from build123d import *

# Parameters (mm, degrees)
SKETCH1_W           = 8.482282434
SKETCH1_H           = 31.931379298
SKETCH1_R           = 3
SKETCH1_W_2         = 15
SKETCH1_H_2         = 6.200324761
SKETCH1_R_2         = 1.425
BOSS_EXTRUDE1_DEPTH = 4
FILLET3_R           = 25
FILLET4_R           = 5


with BuildPart() as part:
    # Sketch1 → Boss-Extrude1 (new body)
    with BuildSketch(Plane.XY):
        with BuildLine():
            ThreePointArc((4.241141217, 39.891935908), (0, 41.554196678), (-4.241141217, 39.891935908))
            Line((-4.241141217, 39.891935908), (-10, 28.882352941))
            Line((-10, 28.882352941), (-10, 0))
            Line((-10, 0), (-25.107692308, 0))
            Line((-25.107692308, 0), (-34, -17))
            Line((-34, -17), (34, -17))
            Line((34, -17), (25.107692308, 0))
            Line((25.107692308, 0), (10, 0))
            Line((10, 0), (10, 28.882352941))
            Line((10, 28.882352941), (4.241141217, 39.891935908))
        make_face()
        with Locations((0, 11.439217567)):
            Rectangle(SKETCH1_W, SKETCH1_H, mode=Mode.SUBTRACT)
        with Locations((0, 33)):
            Circle(SKETCH1_R, mode=Mode.SUBTRACT)
        with Locations((16.5, -5.259184167)):
            Rectangle(SKETCH1_W_2, SKETCH1_H_2, mode=Mode.SUBTRACT)
        with Locations((24, -12)):
            Circle(SKETCH1_R_2, mode=Mode.SUBTRACT)
        with Locations((-24, -12)):
            Circle(SKETCH1_R_2, mode=Mode.SUBTRACT)
        with Locations((-16.5, -5.259184167)):
            Rectangle(SKETCH1_W_2, SKETCH1_H_2, mode=Mode.SUBTRACT)
        with Locations((0, -12)):
            Circle(SKETCH1_R_2, mode=Mode.SUBTRACT)
    extrude(amount=BOSS_EXTRUDE1_DEPTH)

    # Fillet3
    # the kernel refuses this fillet: 25 mm, written as the material it adds along each edge
    with BuildSketch(Plane(origin=(10, 0, 0), x_dir=(1, 0, 0), z_dir=(0, 0, 1))) as fillet3_piece_1:
        with BuildLine():
            CenterArc((25, 22.959578579), FILLET3_R, 180, 66.690841486)
            Line((0, 22.959578579), (-0.5, 22.959578579))
            Line((-0.5, 22.959578579), (-0.5, 0))
            Line((-0.5, 0), (0, -0.5))
            ThreePointArc((0, -0.5), (7.553846154, -0.5), (14.909846154, -0.459191572))
            Line((14.909846154, -0.459191572), (15.107692308, 0))
        make_face()
    extrude(amount=4)
    with BuildSketch(Plane(origin=(-10, 0, 0), x_dir=(0, 1, 0), z_dir=(0, 0, 1))) as fillet3_piece_2:
        with BuildLine():
            CenterArc((22.959578579, 25), FILLET3_R, 203.309158514, 66.690841486)
            Line((0, 15.107692308), (-0.459191572, 14.909846154))
            ThreePointArc((-0.459191572, 14.909846154), (-0.5, 7.553846154), (-0.5, 0))
            Line((-0.5, 0), (0, -0.5))
            Line((0, -0.5), (22.959578579, -0.5))
            Line((22.959578579, -0.5), (22.959578579, 0))
        make_face()
    extrude(amount=4)

    # Fillet4
    # the kernel refuses this fillet: 5 mm, written as the material it adds along each edge
    with BuildSketch(Plane(origin=(4.241141217, -4.526472082, 0), x_dir=(0, 1, 0), z_dir=(0, 0, 1)), Plane(origin=(4.241141217, 27.404907216, 0), x_dir=(-1, 0, 0), z_dir=(0, 0, 1)), Plane(origin=(-24, -2.159021786, 0), x_dir=(0, -1, 0), z_dir=(0, 0, 1)), Plane(origin=(-9, -2.159021786, 0), x_dir=(-1, 0, 0), z_dir=(0, 0, 1)), Plane(origin=(9, -8.359346547, 0), x_dir=(1, 0, 0), z_dir=(0, 0, 1)), Plane(origin=(9, -2.159021786, 0), x_dir=(0, -1, 0), z_dir=(0, 0, 1))) as fillet4_piece_1:
        with BuildLine():
            CenterArc((FILLET4_R, FILLET4_R), FILLET4_R, 180, 90)
            Line((0, FILLET4_R), (0, 0))
            Line((0, 0), (FILLET4_R, 0))
        make_face()
    extrude(amount=4)
    with BuildSketch(Plane(origin=(-4.241141217, -4.526472082, 0), x_dir=(0, 1, 0), z_dir=(0, 0, 1)), Plane(origin=(-4.241141217, 27.404907216, 0), x_dir=(1, 0, 0), z_dir=(0, 0, 1)), Plane(origin=(-24, -8.359346547, 0), x_dir=(0, 1, 0), z_dir=(0, 0, 1)), Plane(origin=(-9, -8.359346547, 0), x_dir=(-1, 0, 0), z_dir=(0, 0, 1)), Plane(origin=(24, -8.359346547, 0), x_dir=(-1, 0, 0), z_dir=(0, 0, 1)), Plane(origin=(24, -2.159021786, 0), x_dir=(0, -1, 0), z_dir=(0, 0, 1))) as fillet4_piece_2:
        with BuildLine():
            CenterArc((FILLET4_R, -FILLET4_R), FILLET4_R, 90, 90)
            Line((0, -FILLET4_R), (0, 0))
            Line((0, 0), (FILLET4_R, 0))
        make_face()
    extrude(amount=4)
    # the kernel refuses this fillet: 5 mm, written as the material it takes off along each edge
    with BuildSketch(Plane(origin=(34, -17, -20.64524995), x_dir=(-1, 0, 0), z_dir=(0, 0, 1)), Plane(origin=(-34, -17, -20.64524995), x_dir=(0.46349752669999783, 0.88609821280882, 0), z_dir=(0, 0, 1))) as fillet4_2_piece_1:
        with BuildLine():
            CenterArc((FILLET4_R * 1.65161999601, -FILLET4_R), FILLET4_R, 90, 117.613027823)
            Line((FILLET4_R * 0.765521783197, -FILLET4_R * 1.4634975267), (0, 0))
            Line((0, 0), (FILLET4_R * 1.65161999601, 0))
        make_face()
    extrude(amount=45.2904999, mode=Mode.SUBTRACT)
    with BuildSketch(Plane(origin=(25.107692308, 0, -4.210996565), x_dir=(-0.9057801330120623, 0.42374798010214837, 0), z_dir=(0, 0, 1))) as fillet4_2_piece_2:
        with BuildLine():
            CenterArc((1.691402393, 4.997635108), FILLET4_R, 232.68446816, 35.553250017)
            Line((-1.339617689, 1.021089212), (0, 0))
            ThreePointArc((0, 0), (0.768819269, 0.011824458), (1.537638539, 0))
        make_face()
    extrude(amount=12.421993131, mode=Mode.SUBTRACT)
    with BuildSketch(Plane(origin=(-25.107692308, 0, -4.210996565), x_dir=(0.9057801330120621, 0.4237479801021487, 0), z_dir=(0, 0, 1))) as fillet4_2_piece_3:
        with BuildLine():
            CenterArc((1.691402393, -4.997635108), FILLET4_R, 91.762281823, 35.553250017)
            Line((-1.339617689, -1.021089212), (0, 0))
            ThreePointArc((0, 0), (0.768819269, -0.011824458), (1.537638539, 0))
        make_face()
    extrude(amount=12.421993131, mode=Mode.SUBTRACT)


solid = part.part
Model file for the job. Use its own axes, mm. A direction names the side the tool comes from. Give positions to 0.01 mm unless a question says otherwise; leave off trailing zeros. Loops run counter-clockwise (first coordinate to the right, second up) from the corner with the lowest first, then second, coordinate; pieces in that order, holes last. Notation, with made-up numbers: (78, -3) -> (128, -3) arc R21 ccw to (128, 22) -> close; hole circle Ø1 at (16, 31). An arc over 180 degrees is marked (long way). Use a Markdown table: item, result. Add a question column.
(1) Slice it at A-A on y = 2.5. List the corners of the cut face in (x, z).
(2) Drop flat-ended pins along their axis: pin 1 Ø2 at (x, z) = (-20, 3.5) entering from +Y; pin 2 Ø1.2 at (y, z) = (17, 1) entering from +X; pin 3 Ø2 at (y, z) = (17, 3) entering from -X. Give the stop position or say it passes through.
(3) Slice it at B-B on y = -7. List the corners of the cut face in (x, z), and give its area (3 significant figures).
(4) Slice it at D-D on y = 33. List the corners of the cut face in (x, z).
(5) Slice it at C-C on z = 1.4. Give the number of separate pieces and of enclosed holes in the cut face, and give its area (3 significant figures).
(6) Wall check: line 1 along X through (y, z) = (-3, 0.85); line 2 along Y through (x, z) = (15.5, 3.3); line 3 along Y through (x, z) = (20, 1.45). Give the ranges that are in metal, low to high.
(7) Tool access for faces 1 (the cylindrical face through (-24.954, -0.235, 1.972)), 2 (the flat face through (4.241, 11, 2)), 3 (the flat face through (10, 26, 2)): list every direction of +Z, -Z, +X, -X, +Y, -Y with a clear straight run to the whole face (end or side of a thin tool).
(8) Mould opens along X. For faces 4 (the cylindrical face through (-21.8, -7.5, 2)), 5 (the flat face through (28.06, -5.64, 1.97)), 6 (the flat face through (16, -2.159, 2)), 7 (the flat face through (-7.08, 34.464, 1.972)) say: +X half, -X half, draft (parallel to the pull), parting line (faces both ways), or undercut.
Filled sheet:
| question | item | result |
|---|---|---|
| 1 | outline | (-20.63, 0) -> (-4.24, 0) -> (-4.24, 4) -> (-20.63, 4) -> close; (4.24, 0) -> (20.63, 0) -> (20.63, 4) -> (4.24, 4) -> close |
| 2 | pin 1 | y = 3.75 |
| 2 | pin 2 | x = 10.88 |
| 2 | pin 3 | x = -10.99 |
| 3 | outline | (-28.77, 0) -> (-22.43, 0) -> (-22.43, 4) -> (-28.77, 4) -> close; (-10.57, 0) -> (10.57, 0) -> (10.57, 4) -> (-10.57, 4) -> close; (22.43, 0) -> (28.77, 0) -> (28.77, 4) -> (22.43, 4) -> close |
| 3 | area | 135 mm2 |
| 4 | outline | (-7.85, 0) -> (-3, 0) -> (-3, 4) -> (-7.85, 4) -> close; (3, 0) -> (7.85, 0) -> (7.85, 4) -> (3, 4) -> close |
| 5 | separate pieces | 1 |
| 5 | enclosed holes | 7 |
| 5 | area | 1,470 mm2 |
| 6 | line 1 | -26.68 to -21.78, -11.22 to -2.84, 2.84 to 11.22, 21.78 to 26.68 |
| 6 | line 2 | -17 to -8.36, -2.16 to 7.32 |
| 6 | line 3 | -17 to -8.26, -2.26 to 2.96 |
| 7 | face 1 | +Z, -Z, -X, +Y |
| 7 | face 2 | +Z, -Z |
| 7 | face 3 | +Z, -Z, +X, +Y |
| 8 | face 4 | undercut |
| 8 | face 5 | +X half |
| 8 | face 6 | undercut |
| 8 | face 7 | -X half |
